Part model, mm, in its own coordinate system. Round coordinates to 2 decimals unless told otherwise and drop trailing zeros. Write each loop counter-clockwise with the first axis right and the second up, starting at its lowest first coordinate (ties: lowest second). Pieces come first, ordered by that corner, then holes.
1) Saw through at D-D on z = 1.1. Write the cut outline in (x, y), and give its area (3 significant figures).
2) Saw through at B-B on y = -35.5. Write the cut outline in (x, z), and give its area (3 significant figures).
3) Flat gauge pin, fed straight in: pin 1 (2.5 mm diameter, centred on x = 42.82, y = -44.47, fed in from -Z). Where does the tip first touch, or does it go through?
4) Drill centre lines: L1, parallel to Y at x = 43, z = 0.85; L2, parallel to X at y = -29, z = 2.5; L3, parallel to Y at x = 44, z = 0.35. Where is each one in solid material? Low to high.
5) Saw through at C-C on y = -44. Write the cut outline in (x, z).
6) Saw through at A-A on x = 54. Write the cut outline in (y, z).
Autodesk Inventor part; units mm, degrees
ref_plane "YZ Plane" through (0, 0, 0) normal (1, 0, 0) x (0, 1, 0)
ref_plane "XZ Plane" through (0, 0, 0) normal (0, 1, 0) x (-1, 0, 0)
ref_plane "XY Plane" through (0, 0, 0) normal (0, 0, 1) x (1, 0, 0)
sketch "Szkic1" plane through (0, 0, 0) normal (0, 0, 1) x (1, 0, 0)
  line L0 (37.3233, -49.9659) -> (79.3233, -49.9659)
  line L1 (79.3233, -49.9659) -> (79.3233, -7.9659)
  line L2 (79.3233, -7.9659) -> (37.3233, -7.9659)
  line L3 (37.3233, -49.9659) -> (37.3233, -7.9659)
  point P0 (0, 0)
  point P1 (42.8233, -13.4659)
  point P2 (73.8233, -13.4659)
  point P3 (42.8233, -44.4659)
  point P4 (73.8233, -44.4659)
  point P5 (58.3233, -28.9659)
  dimension "d0" = 42
  dimension "d2" = 15.5
  dimension "d3" = 15.5
  dimension "d4" = 15.5
  dimension "d5" = 15.5
  dimension "d6" = 15.5
  dimension "d7" = 15.5
  dimension "d8" = 15.5
  dimension "d9" = 15.5
  dimension "d10" = 21
  dimension "d11" = 21
  dimension "d19" = 21
extrude "Wyciągnięcie proste1" add sketch "Szkic1" along normal blind 3
hole "Otwór1" at (73.8233, -44.4659, 0) at (42.8233, -44.4659, 0) at (73.8233, -13.4659, 0) at (42.8233, -13.4659, 0) direction (0, 0, 1) diameter 3 end through all
hole "Otwór2" at (58.3233, -28.9659, 0) direction (0, 0, 1) diameter 22.5 end through all
chamfer "Faza1" distance 2 angle 45 4 edges at (37.3233, -7.9659, 1.5) (79.3233, -7.9659, 1.5) (79.3233, -49.9659, 1.5) (37.3233, -49.9659, 1.5)
properties part number "3DP_ABS_X_Axis_Motor_Spacer"
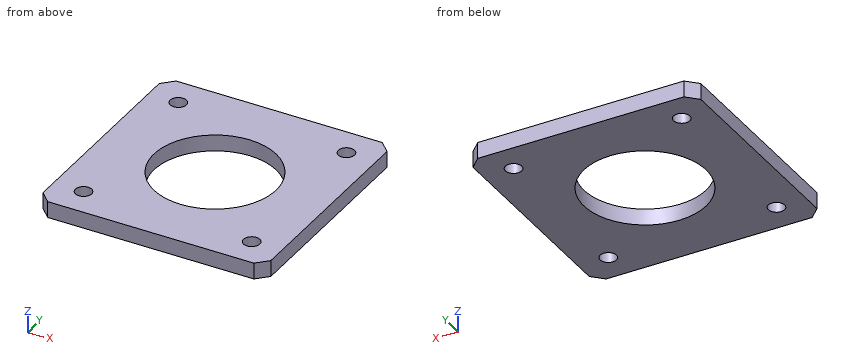
Completed:
1. outline: (37.32, -47.97) - (39.32, -49.97) - (77.32, -49.97) - (79.32, -47.97) - (79.32, -9.97) - (77.32, -7.97) - (39.32, -7.97) - (37.32, -9.97) - close; hole circle Ø3 at (42.82, -44.47); hole circle Ø3 at (42.82, -13.47); hole circle Ø22.5 at (58.32, -28.97); hole circle Ø3 at (73.82, -44.47); hole circle Ø3 at (73.82, -13.47)
1. area: 1,330 mm2
2. outline: (37.32, 0) - (49.17, 0) - (49.17, 3) - (37.32, 3) - close; (67.48, 0) - (79.32, 0) - (79.32, 3) - (67.48, 3) - close
2. area: 71.1 mm2
3. pin 1: passes through
4. L1: y = -49.97 to -45.96, -42.98 to -14.96, -11.98 to -7.97
4. L2: x = 37.32 to 47.07, 69.57 to 79.32
4. L3: y = -49.97 to -45.4, -43.54 to -14.4, -12.54 to -7.97
5. outline: (37.32, 0) - (41.4, 0) - (41.4, 3) - (37.32, 3) - close; (44.25, 0) - (72.4, 0) - (72.4, 3) - (44.25, 3) - close; (75.25, 0) - (79.32, 0) - (79.32, 3) - (75.25, 3) - close
6. outline: (-49.97, 0) - (-39.35, 0) - (-39.35, 3) - (-49.97, 3) - close; (-18.58, 0) - (-7.97, 0) - (-7.97, 3) - (-18.58, 3) - close
